Check sheet for the modelled part. Datum: model origin and axes. Units: mm. Face numbers are marked on the shaded views. Give positions to 0.01 mm unless a question says otherwise; leave off trailing zeros. Order: outer loops, then holes, each group sorted by start corner. A loop starts at its lowest first (then second) coordinate and runs counter-clockwise, first axis right, second up.
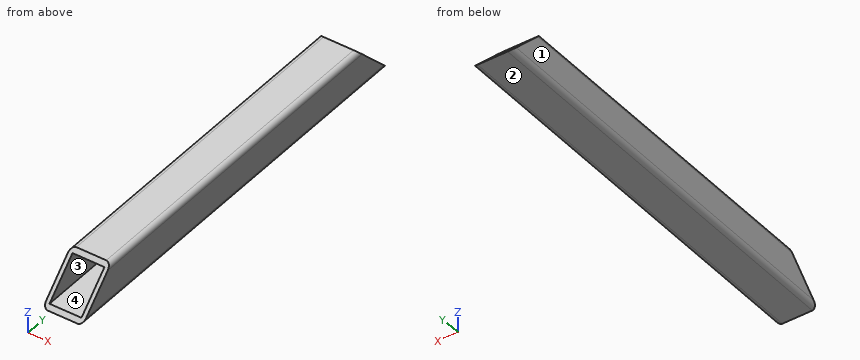
```python
from build123d import *

# Parameters (mm, degrees)
F0_W     = 32
F0_H     = 32
F1_DEPTH = 424.264
F2_W     = 32
F2_H     = 32
F3_ANGLE = 45
F4_W     = 32
F4_H     = 32
F5_ANGLE = 45


with BuildPart() as f1:
    # F0 (on Front) → F1 (new body)
    with BuildSketch(Plane.XZ):
        with BuildLine():
            Line((-15, -20), (15, -20))
            ThreePointArc((15, -20), (18.5355339059, -18.5355339059), (20, -15))
            Line((20, -15), (20, 15))
            ThreePointArc((20, 15), (18.5355339059, 18.5355339059), (15, 20))
            Line((15, 20), (-15, 20))
            ThreePointArc((-15, 20), (-18.5355339059, 18.5355339059), (-20, 15))
            Line((-20, 15), (-20, -15))
            ThreePointArc((-20, -15), (-18.5355339059, -18.5355339059), (-15, -20))
        make_face()
        Rectangle(F0_W, F0_H, mode=Mode.SUBTRACT)
    extrude(amount=F1_DEPTH)

    # F2 (on face) → F3 (revolve, cut)
    with BuildSketch(Plane.XZ.offset(424.264)):
        with BuildLine():
            Line((-15, -20), (15, -20))
            ThreePointArc((15, -20), (18.5355339059, -18.5355339059), (20, -15))
            Line((20, -15), (20, 15))
            ThreePointArc((20, 15), (18.5355339059, 18.5355339059), (15, 20))
            Line((15, 20), (-15, 20))
            ThreePointArc((-15, 20), (-18.5355339059, 18.5355339059), (-20, 15))
            Line((-20, 15), (-20, -15))
            ThreePointArc((-20, -15), (-18.5355339059, -18.5355339059), (-15, -20))
        make_face()
        Rectangle(F2_W, F2_H, mode=Mode.SUBTRACT)
        with BuildLine():
            ThreePointArc((15, 20), (18.5355339059, 18.5355339059), (20, 15))
            Line((20, 15), (20, 20))
            Line((20, 20), (15, 20))
        make_face()
        with BuildLine():
            Line((-20, 20), (-20, 15))
            ThreePointArc((-20, 15), (-18.5355339059, 18.5355339059), (-15, 20))
            Line((-15, 20), (-20, 20))
        make_face()
        with BuildLine():
            Line((15, -20), (20, -20))
            Line((20, -20), (20, -15))
            ThreePointArc((20, -15), (18.5355339059, -18.5355339059), (15, -20))
        make_face()
        Rectangle(F2_W, F2_H)
        Polygon((15, 20), (20, 20), (20, 37), (-20, 37), (-20, 20), (-15, 20), align=None)
        with BuildLine():
            Line((-20, -20), (-15, -20))
            ThreePointArc((-15, -20), (-18.5355339059, -18.5355339059), (-20, -15))
            Line((-20, -15), (-20, -20))
        make_face()
    revolve(axis=Axis((0, -424.264, -20), (-1, 0, 0)), revolution_arc=F3_ANGLE, mode=Mode.SUBTRACT)

    # F4 (on face) → F5 (revolve, cut)
    with BuildSketch(Plane(origin=(0, 0, 0), x_dir=(-1, 0, 0), z_dir=(0, 1, 0))):
        with BuildLine():
            ThreePointArc((-20, -15), (-18.5355339059, -18.5355339059), (-15, -20))
            Line((-15, -20), (15, -20))
            ThreePointArc((15, -20), (18.5355339059, -18.5355339059), (20, -15))
            Line((20, -15), (20, 15))
            ThreePointArc((20, 15), (18.5355339059, 18.5355339059), (15, 20))
            Line((15, 20), (-15, 20))
            ThreePointArc((-15, 20), (-18.5355339059, 18.5355339059), (-20, 15))
            Line((-20, 15), (-20, -15))
        make_face()
        Rectangle(F4_W, F4_H, mode=Mode.SUBTRACT)
        Rectangle(F4_W, F4_H)
        with BuildLine():
            Line((-20, 37), (-20, 15))
            ThreePointArc((-20, 15), (-18.5355339059, 18.5355339059), (-15, 20))
            Line((-15, 20), (15, 20))
            ThreePointArc((15, 20), (18.5355339059, 18.5355339059), (20, 15))
            Line((20, 15), (20, 37))
            Line((20, 37), (-20, 37))
        make_face()
        with BuildLine():
            ThreePointArc((20, -15), (18.5355339059, -18.5355339059), (15, -20))
            Line((15, -20), (20, -20))
            Line((20, -20), (20, -15))
        make_face()
        with BuildLine():
            Line((-20, -15), (-20, -20))
            Line((-20, -20), (-15, -20))
            ThreePointArc((-15, -20), (-18.5355339059, -18.5355339059), (-20, -15))
        make_face()
    revolve(axis=Axis((0, 0, -20), (1, 0, 0)), revolution_arc=F5_ANGLE, mode=Mode.SUBTRACT)


solid = f1.part
```
(1) Cross-section at B-B on y = -363. Enter the section's corners in (x, z).
Response values:
outline: (-20, -15) arc R5 ccw to (-15, -20) - (15, -20) arc R5 ccw to (20, -15) - (20, 15) arc R5 ccw to (15, 20) - (-15, 20) arc R5 ccw to (-20, 15) - close; hole (-16, -16) - (16, -16) - (16, 16) - (-16, 16) - close
(2) Cross-section at C-C on z = -5. Enter the section's corners in (x, y).
Response values:
outline: (-20, -409.26) - (-16, -409.26) - (-16, -15) - (-20, -15) - close; (16, -409.26) - (20, -409.26) - (20, -15) - (16, -15) - close
(3) Release check for a two-part mould opening along X. For the marked faces 1, 2, 3 and 4 record: released by +X, released by -X, zero draft, split by the parting line, or undercut.
Response values:
face 1: released by -X
face 2: zero draft
face 3: undercut
face 4: undercut
(4) Cross-section at A-A on x = -3. Enter the section's corners in (y, z), then the cut area to 3 significant figures.
Response values:
outline: (-424.26, -20) - (0, -20) - (-4, -16) - (-420.26, -16) - close; (-388.26, 16) - (-36, 16) - (-40, 20) - (-384.26, 20) - close
area: 3,070 mm2
(5) Material ranges on L1, parallel to X at y = -104, z = 1.5; L2, parallel to Z at x = -14, y = -403.5, recorded low to high.
Response values:
L1: x = -20 to -16, 16 to 20
L2: z = -20 to -16
(6) Gauge pin test, flat ends, axial feed: pin 1 Ø8 at (x, z) = (9, -11) entering from +Y; pin 2 Ø12 at (x, z) = (1.5, -13) entering from +Y. Record the tip position at first contact, or that the pin passes through.
Response values:
pin 1: passes through
pin 2: stops at y = -1
